Design review of the part built by this model. Coordinates are the model's own, in mm. A direction names the side the tool comes from. Round coordinates to 2 decimals unless told otherwise and drop trailing zeros. Order: outer loops, then holes, each group sorted by start corner. A loop starts at its lowest first (then second) coordinate and runs counter-clockwise, first axis right, second up.
from build123d import *

# Parameters (mm, degrees)
SKETCH1_R           = 18.4
BOSS_EXTRUDE1_DEPTH = 67.6
SKETCH2_R           = 6
BOSS_EXTRUDE2_DEPTH = 6
BOSS_EXTRUDE3_START = -6
BOSS_EXTRUDE3_DEPTH = 22


with BuildPart() as part:
    # Sketch1 → Boss-Extrude1 (new body)
    with BuildSketch(Plane(origin=(0, 0, 0), x_dir=(1, 0, 0), z_dir=(0, 1, 0))):
        with Locations(Location((0, 0, 0), (0, 0, 270))):
            Circle(SKETCH1_R)
    extrude(amount=BOSS_EXTRUDE1_DEPTH)

    # Sketch2 → Boss-Extrude2 (add)
    with BuildSketch(Plane(origin=(0, 67.6, 0), x_dir=(1, 0, 0), z_dir=(0, 1, 0))):
        with Locations(Location((0, -7, 0), (0, 0, 270))):
            Circle(SKETCH2_R)
    extrude(amount=BOSS_EXTRUDE2_DEPTH)

    # Sketch3 → Boss-Extrude3 (add)
    with BuildSketch(Plane(origin=(0, 73.6, 0), x_dir=(1, 0, 0), z_dir=(0, 1, 0)).offset(BOSS_EXTRUDE3_START)):
        with BuildLine():
            Line((-1.697056275, -4.9), (1.697056275, -4.9))
            ThreePointArc((1.697056275, -4.9), (0, -9.7), (-1.697056275, -4.9))
        make_face()
    extrude(amount=BOSS_EXTRUDE3_DEPTH)


solid = part.part
1) Take a section at C-C on y = 8. Give the boundary of the cut face in (x, z), plus the area to 3 significant figures.
Results:
outline: circle Ø36.8 at (0, 0)
area: 1,060 mm2
2) Take a section at D-D on z = 0. Give the boundary of the cut face in (x, y), plus the area to 3 significant figures.
Results:
outline: (-18.4, 0) - (18.4, 0) - (18.4, 67.6) - (-18.4, 67.6) - close
area: 2,490 mm2
3) To check wall thickness, follow line 1 along Y through (x, z) = (3, -15); line 2 along X through (y, z) = (4, -0.5); line 3 along Z through (x, y) = (-14.5, 13). State the ranges of each line that lie inside material, in increasing order.
Results:
line 1: y = 0 to 67.6
line 2: x = -18.39 to 18.39
line 3: z = -11.33 to 11.33
4) For faces 1 (the face through (0, 81, 4.9)), 2 (the face through (0, 89.6, 7)), 3 (the face through (0.1, 81.5, 9.7)), list the 3-axis set-ups (+Z, -Z, +X, -X, +Y, -Y) from which the entire face can be reached by the end or side of a thin tool; tool diameter is ignored.
Results:
face 1: -Z, +X, -X, +Y
face 2: +Z, -Z, +X, -X, +Y
face 3: +Y
5) Clearance check with flat-ended pins moving along their axes: P1, Ø1, axis at x = 0, y = 82, coming from the -Z side; P2, Ø12, axis at y = 45.5, z = -4, coming from the +X side; P3, Ø3, axis at y = 47.5, z = 11, coming from the +X side. State where each tip first meets the part, or that it passes through.
Results:
P1: stops at z = 4.9
P2: stops at x = 18.4
P3: stops at x = 15.76
6) Take a section at B-B on z = 7. Give the boundary of the cut face in (x, y).
Results:
outline: (-17.02, 0) - (17.02, 0) - (17.02, 67.6) - (6, 67.6) - (6, 73.6) - (2.7, 73.6) - (2.7, 89.6) - (-2.7, 89.6) - (-2.7, 73.6) - (-6, 73.6) - (-6, 67.6) - (-17.02, 67.6) - close
7) Take a section at A-A on x = 0. Give the boundary of the cut face in (y, z), plus the area to 3 significant figures.
Results:
outline: (0, -18.4) - (67.6, -18.4) - (67.6, 1) - (73.6, 1) - (73.6, 4.9) - (89.6, 4.9) - (89.6, 9.7) - (73.6, 9.7) - (73.6, 13) - (67.6, 13) - (67.6, 18.4) - (0, 18.4) - close
area: 2,640 mm2
